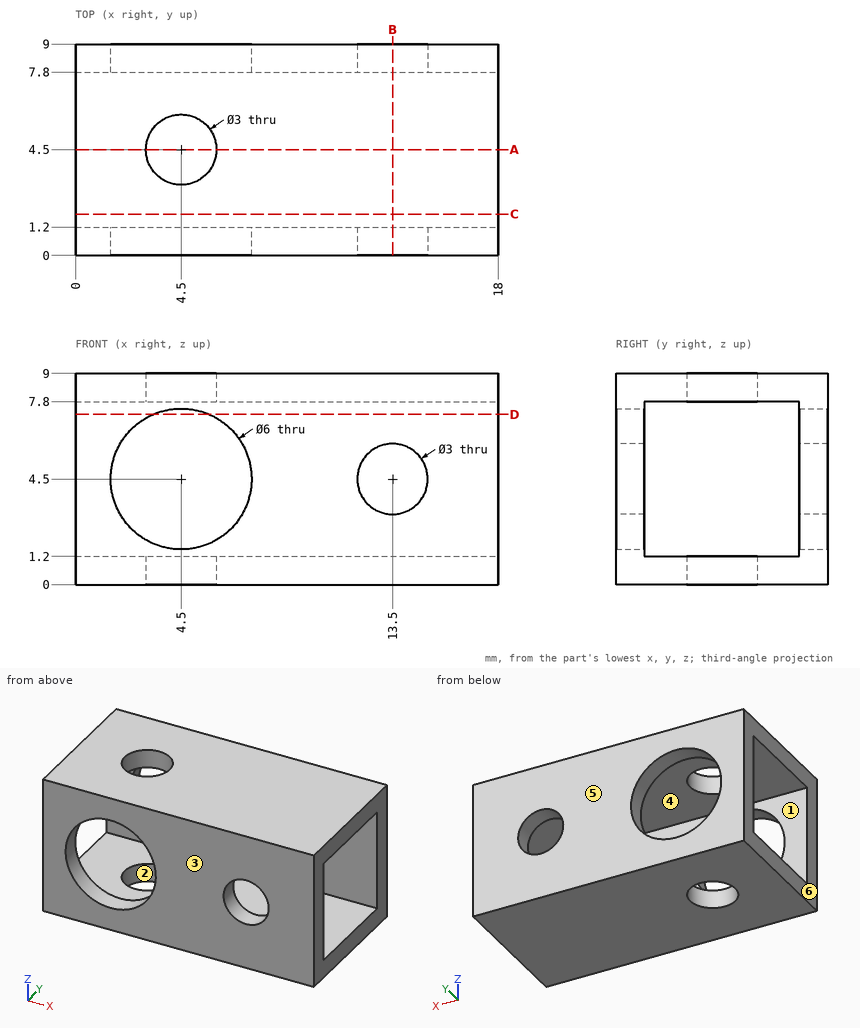
Design review of the part shown in the three views and the two pictorial views. Dimensions are in mm from the part's minimum x, y and z. A direction names the side the tool comes from. Round coordinates to 2 decimals unless told otherwise and drop trailing zeros. Loops run counter-clockwise (first coordinate to the right, second up) from the corner with the lowest first, then second, coordinate; pieces in that order, holes last.
1) The part is to be moulded in two halves that separate along Y. For the marked faces 3, 4, 5 and 6, say which applies: pulls with the +Y half, pulls with the -Y half, needs draft (parallel to the pull), parting line crosses it, or undercut.
Values follow:
face 3: pulls with the -Y half
face 4: undercut
face 5: pulls with the +Y half
face 6: needs draft
2) Tool access review of the marked faces 1 and 2: name each direction out of +Z, -Z, +X, -X, +Y, -Y from which nothing blocks a thin tool from reaching the whole face with its end or side.
Values follow:
face 1: +X, -X
face 2: +Z, -Z
3) Consider section B-B on x = 13.5. State the section outline as (y, z) points, then the cut area to 3 significant figures.
Values follow:
outline: (0, 0) - (9, 0) - (9, 3) - (7.8, 3) - (7.8, 1.2) - (1.2, 1.2) - (1.2, 3) - (0, 3) - close; (0, 6) - (1.2, 6) - (1.2, 7.8) - (7.8, 7.8) - (7.8, 6) - (9, 6) - (9, 9) - (0, 9) - close
area: 30.2 mm2
4) Clearance check with flat-ended pins moving along their axes: P1, Ø1.8, axis at x = 13.5, z = 4.5, coming from the +Y side; P2, Ø3, axis at y = 7.5, z = 3.5, coming from the -X side. State where each tip first meets the part, or that it passes through.
Values follow:
P1: passes through
P2: stops at x = 0
5) Consider section A-A on y = 4.5. State the section outline as (x, z) points, then the cut area to 3 significant figures.
Values follow:
outline: (0, 0) - (3, 0) - (3, 1.2) - (0, 1.2) - close; (0, 7.8) - (3, 7.8) - (3, 9) - (0, 9) - close; (6, 0) - (18, 0) - (18, 1.2) - (6, 1.2) - close; (6, 7.8) - (18, 7.8) - (18, 9) - (6, 9) - close
area: 36.0 mm2
6) Wall thickness on line 1 along X through (y, z) = (0.95, 4.5); line 2 along Y through (x, z) = (4.5, 8.7); line 3 along Z through (x, y) = (7.75, 4.25): over which ranges is each line inside the solid? List them lowest first.
Values follow:
line 1: x = 0 to 1.5, 7.5 to 12, 15 to 18
line 2: y = 0 to 3, 6 to 9
line 3: z = 0 to 1.2, 7.8 to 9
7) Consider section D-D on z = 7.25. State the section outline as (x, y) points, then the cut area to 3 significant figures.
Values follow:
outline: (0, 0) - (3.3, 0) - (3.3, 1.2) - (0, 1.2) - close; (0, 7.8) - (3.3, 7.8) - (3.3, 9) - (0, 9) - close; (5.7, 0) - (18, 0) - (18, 1.2) - (5.7, 1.2) - close; (5.7, 7.8) - (18, 7.8) - (18, 9) - (5.7, 9) - close
area: 37.4 mm2
8) Consider section C-C on y = 1.75. State the section outline as (x, z) points.
Values follow:
outline: (0, 0) - (18, 0) - (18, 1.2) - (0, 1.2) - close; (0, 7.8) - (18, 7.8) - (18, 9) - (0, 9) - close
